Input: part model. Units: mm. Frame: model coordinates. A direction names the side the tool comes from. Round coordinates to 2 decimals unless told otherwise and drop trailing zeros. Order: outer loops, then holes, each group sorted by start corner. A loop starts at its lowest first (then second) coordinate and runs counter-clockwise, first axis right, second up. Notation, with made-up numbers: (52, 67.25) -> (83, 67.25) arc R12 ccw to (83, 86.25) -> close; hole circle Ø7 at (34.25, -7). An arc over 180 degrees is marked (long way). Answer as CSV lines item,"result". Start each with the question number.
1) First-contact query: P1, Ø4, axis at x = -23.5, y = 0, coming from the +Z side; P2, Ø2, axis at x = -2, z = 10, coming from the +Y side; P3, Ø1.5, axis at y = 7.5, z = 5, coming from the +X side. Flat tips, straight axial feed; report the tip coordinate or a pass-through.
2) Mould query, pull axis Y, two halves, no side actions, for faces 1 (the face through (-29.97, 1.32, 2.46)), 2 (the face through (13, 0, 0)), 3 (the face through (-19, 0, 2)). Classes: +Y half, -Y half, draft (parallel to the pull), parting line (faces both ways), or undercut.
3) Line query: L1, parallel to Z at x = -18.5, y = 12.5; L2, parallel to X at y = 6, z = 9.5; L3, parallel to Y at x = 0, z = 9.75. Output: solid intervals per line, ascending.
4) Section query C-C, the plane x = -22. Output: boundary loops of the cut face in (y, z), and give its area (3 significant figures).
5) Access query for faces 4 (the face through (0, -19, 2)), 5 (the face through (-14.985, 0.66, 8.451)). Directions: +Z, -Z, +X, -X, +Y, -Y. A direction counts if a zero-diameter tool reaches every point of the face in a straight line with its end or side. Return the directions, or none.
6) Section query A-A, the plane x = 0. Output: boundary loops of the cut face in (y, z), and give its area (3 significant figures).
7) Section query D-D, the plane z = 9. Output: boundary loops of the cut face in (x, y).
```python
from build123d import *

# Parameters (mm, degrees)
CYLINDER003_R     = 3
CYLINDER003_DEPTH = 10
ARRAY_COUNT       = 8
CYLINDER002_R     = 10
CYLINDER002_DEPTH = 30
CYLINDER001_R     = 15
CYLINDER001_DEPTH = 12
CYLINDER_R        = 30
CYLINDER_DEPTH    = 5


with BuildPart() as array:
    # Cylinder003 → Cylinder003 (new body)
    with BuildSketch(Plane(origin=(22, 0, -2), x_dir=(1, 0, 0), z_dir=(0, 0, 1))):
        Circle(CYLINDER003_R)
    extrude(amount=CYLINDER003_DEPTH)

    # Array: Array ×8 about axis
    array_axis = Axis((0, 0, 0), (0, 0, 1))


with BuildPart() as array_1:
    add(array.part)
    for i in range(1, ARRAY_COUNT):
        add(array.part.rotate(array_axis, i * 360 / ARRAY_COUNT))


with BuildPart() as cilindro:
    # Cylinder002 → Cylinder002 (new body)
    with BuildSketch(Plane.XY.offset(-2)):
        Circle(CYLINDER002_R)
    extrude(amount=CYLINDER002_DEPTH)


with BuildPart() as tubo_exterior:
    # Cylinder001 → Cylinder001 (new body)
    with BuildSketch(Plane.XY):
        Circle(CYLINDER001_R)
    extrude(amount=CYLINDER001_DEPTH)


with BuildPart() as cut001:
    # Cylinder → Cylinder (new body)
    with BuildSketch(Plane.XY):
        Circle(CYLINDER_R)
    extrude(amount=CYLINDER_DEPTH)

    # Fusion: union tubo exterior
    add(tubo_exterior.part)

    # Cut: cut Cilindro
    add(cilindro.part, mode=Mode.SUBTRACT)

    # Cut001: cut Array
    add(array_1.part, mode=Mode.SUBTRACT)


solid = cut001.part
```
Findings:
1,P1,"stops at z = 5"
1,P2,"stops at y = 14.97"
1,P3,"stops at x = 29.23"
2,face 1,"parting line"
2,face 2,"draft"
2,face 3,"undercut"
3,L1,"z = 0 to 5"
3,L2,"x = -13.75 to -8, 8 to 13.75"
3,L3,"y = -15 to -10, 10 to 15"
4,outline,"(-20.4, 0) -> (-3, 0) -> (-3, 5) -> (-20.4, 5) -> close; (3, 0) -> (20.4, 0) -> (20.4, 5) -> (3, 5) -> close"
4,area,"174 mm^2"
5,face 4,"+Z, -Z"
5,face 5,"+Z"
6,outline,"(-30, 0) -> (-25, 0) -> (-25, 5) -> (-30, 5) -> close; (-19, 0) -> (-10, 0) -> (-10, 12) -> (-15, 12) -> (-15, 5) -> (-19, 5) -> close; (10, 0) -> (19, 0) -> (19, 5) -> (15, 5) -> (15, 12) -> (10, 12) -> close; (25, 0) -> (30, 0) -> (30, 5) -> (25, 5) -> close"
6,area,"210 mm^2"
7,outline,"circle Ø30 at (0, 0); hole circle Ø20 at (0, 0)"
